Part print with two shaded views. Sizes in mm from the minimum x, y, z corner. Coordinates: 2 decimals unless noted, no trailing zeros. Write each loop counter-clockwise with the first axis right and the second up, starting at its lowest first coordinate (ties: lowest second). Pieces come first, ordered by that corner, then holes. Notation, with made-up numbers: M 73.25,27.5 L 127.25,27.5 A25 ccw 127.25,58.5 Z; hole C 16,42 d7. An arc over 180 degrees is marked long. One line per question, with ' | ' between items. Start each with the question number.
(1) Cut at A-A (y = 7.75). Write the cut outline in (x, z), plus the area to 3 significant figures.
(2) Cut at C-C (x = 42.5). Write the cut outline in (y, z).
(3) Cut at D-D (y = 3.5). Write the cut outline in (x, z).
(4) Flat gauge pins, fed straight in: pin 1 Ø1.5 at (x, y) = (12.5, 6) entering from +Z; pin 2 Ø2 at (x, y) = (25, 2.5) entering from -Z; pin 3 Ø0.8 at (x, z) = (1.5, 7) entering from -Y; pin 4 Ø6 at (x, z) = (44.5, 5.5) entering from -Y. Where does each tip first touch, or does it go through?
(5) Two-plate mould, pull along X, no slides. Class the marked faces 1, 2, 3 and 4: +X half, -X half, draft (parallel to the pull), parting line (faces both ways), or undercut.
(6) Cut at B-B (z = 7.25). Write the cut outline in (x, y).
(7) Wall check: probe 1 along X at (y, z) = (7.5, 7); probe 2 along X at (y, z) = (4, 5); probe 3 along Y at (x, z) = (27.5, 3.25). Give the ranges that are in metal, low to high.
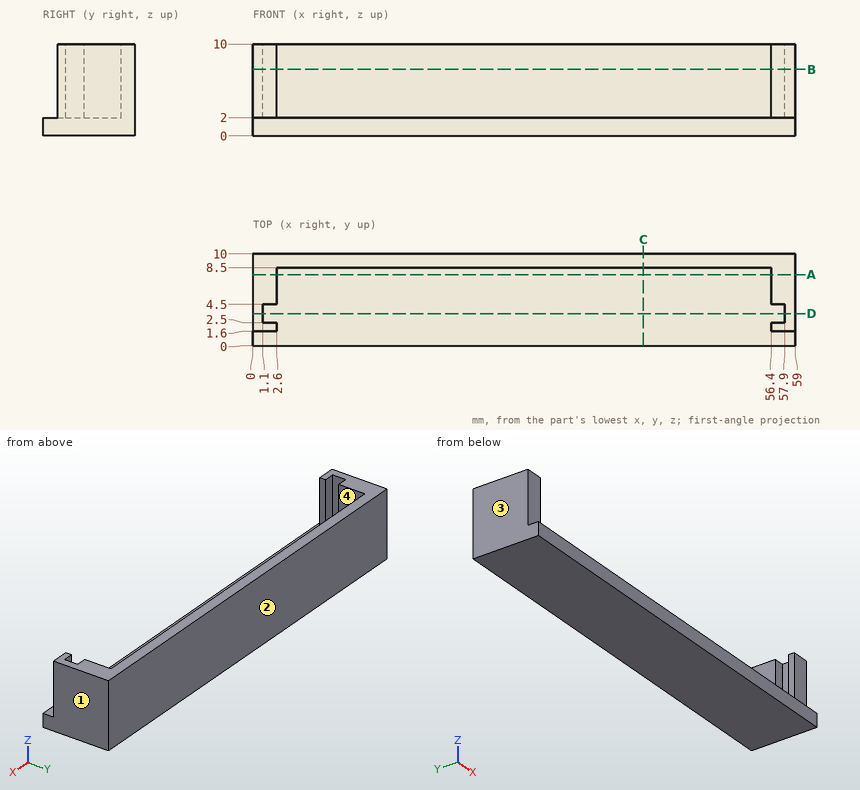
Filled in:
1) outline: M 0,0 L 59,0 L 59,10 L 56.4,10 L 56.4,2 L 2.6,2 L 2.6,10 L 0,10 Z | area: 160 mm²
2) outline: M 0,0 L 10,0 L 10,10 L 8.5,10 L 8.5,2 L 0,2 Z
3) outline: M 0,0 L 59,0 L 59,10 L 57.9,10 L 57.9,2 L 1.1,2 L 1.1,10 L 0,10 Z
4) pin 1: z = 2 | pin 2: z = 0 | pin 3: y = 1.6 | pin 4: y = 8.5
5) face 1: +X half | face 2: draft | face 3: -X half | face 4: undercut
6) outline: M 0,1.6 L 2.6,1.6 L 2.6,2.5 L 1.1,2.5 L 1.1,4.5 L 2.6,4.5 L 2.6,8.5 L 56.4,8.5 L 56.4,4.5 L 57.9,4.5 L 57.9,2.5 L 56.4,2.5 L 56.4,1.6 L 59,1.6 L 59,10 L 0,10 Z
7) probe 1: 0 to 2.6, 56.4 to 59 | probe 2: 0 to 1.1, 57.9 to 59 | probe 3: 8.5 to 10
